Source: CAD feature listing. Evaluate the final solid. Frame: model axes, mm. A direction names the side the tool comes from. Coordinates: 2 decimals unless noted, no trailing zeros.
Item 1: Reachability of faces 1 (the flat face through (-3, -9.525, -1)), 2 (the cylindrical face through (-219.957, -9.18, 24.349)) from +Z, -Z, +X, -X, +Y, -Y: full face, straight path, thin tool, end or side. Return the list, or none.
Item 2: Line query: probe 1 along Z at (x, y) = (215, -3.75); probe 2 along X at (y, z) = (-2.75, 0) (1 decimal); probe 3 along X at (y, z) = (-4.5, 20) (3 decimals). Output: solid intervals per line, ascending.
Item 3: Pin query (flat end, axial travel): pin 1 Ø2.5 at (x, z) = (-216.5, 2.5) entering from -Y. Return the tip coordinate at first contact, or that it passes through.
```python
from build123d import *

# Parameters (mm, degrees)
RESSALTO_EXTRUS_O1_DEPTH        = 9.525
ESBO_O5_R                       = 2.78
CORTE_EXTRUS_O2_DEPTH           = 10
ESBO_O8_R                       = 2.75
CORTE_EXTRUS_O4_DEPTH           = 10
ESBO_O9_R                       = 5
CORTE_EXTRUS_O5_DEPTH           = 0.7
ESBO_O10_R                      = 5
CORTE_EXTRUS_O6_DEPTH           = 2.5
CORTE_EXTRUS_O6_DRAFT           = -45
CORTE_EXTRUS_O6_PROFILE_2_DEPTH = 2.5
CORTE_EXTRUS_O6_PROFILE_2_DRAFT = -45
CORTE_EXTRUS_O6_PROFILE_3_DEPTH = 2.5
CORTE_EXTRUS_O6_PROFILE_3_DRAFT = -45
CORTE_EXTRUS_O6_PROFILE_4_DEPTH = 2.5
CORTE_EXTRUS_O6_PROFILE_4_DRAFT = -45
CORTE_EXTRUS_O6_PROFILE_5_DEPTH = 2.5
CORTE_EXTRUS_O6_PROFILE_5_DRAFT = -45
CORTE_EXTRUS_O6_PROFILE_6_DEPTH = 2.5
CORTE_EXTRUS_O6_PROFILE_6_DRAFT = -45
ESBO_O11_R                      = 2.5
CORTE_EXTRUS_O7_DEPTH           = 10


with BuildPart() as part:
    # Esboço3 → Ressalto-extrusão1 (new body)
    with BuildSketch(Plane(origin=(0, 0, 0), x_dir=(1, 0, 0), z_dir=(0, 1, 0))):
        Polygon((-183.495, 37.21932618), (-246.505, 50), (-246.505, -50), (-183.495, -50), align=None)
        Polygon((-183.495, 50), (-183.495, 37.21932618), (183.495, -37.21932618), (183.495, 50), align=None)
        Polygon((183.495, -37.21932618), (-183.495, 37.21932618), (-183.495, -50), (183.495, -50), align=None)
        Polygon((246.505, -50), (183.495, -37.21932618), (183.495, -50), align=None)
        Polygon((183.495, 50), (183.495, -37.21932618), (246.505, -50), (246.505, 50), align=None)
        Polygon((-183.495, 50), (-246.505, 50), (-183.495, 37.21932618), align=None)
    extrude(amount=-RESSALTO_EXTRUS_O1_DEPTH)

    # Esboço5 → Corte-extrusão2 (cut)
    with BuildSketch(Plane(origin=(0, 0, 0), x_dir=(1, 0, 0), z_dir=(0, 1, 0))):
        with Locations(Location((0, -45.235, 0), (0, 0, 270))):
            Circle(ESBO_O5_R)
        with Locations(Location((-20, -45.235, 0), (0, 0, 270))):
            Circle(ESBO_O5_R)
        with Locations(Location((20, -45.235, 0), (0, 0, 270))):
            Circle(ESBO_O5_R)
        with Locations(Location((-20, 45.235, 0), (0, 0, 270))):
            Circle(ESBO_O5_R)
        with Locations(Location((20, 45.235, 0), (0, 0, 270))):
            Circle(ESBO_O5_R)
        with Locations(Location((0, 45.235, 0), (0, 0, 270))):
            Circle(ESBO_O5_R)
    extrude(amount=-CORTE_EXTRUS_O2_DEPTH, mode=Mode.SUBTRACT)

    # Esboço8 → Corte-extrusão4 (cut)
    with BuildSketch(Plane.XZ.offset(9.525)):
        with Locations(Location((-188.84, 19.950903247, 0), (0, 0, 270))):
            Circle(ESBO_O8_R)
        with Locations(Location((-188.84, -19.95, 0), (0, 0, 270))):
            Circle(ESBO_O8_R)
        with Locations(Location((-241.16, 19.950903247, 0), (0, 0, 270))):
            Circle(ESBO_O8_R)
        with Locations(Location((-241.16, -19.95, 0), (0, 0, 270))):
            Circle(ESBO_O8_R)
        with Locations(Location((241.16, -19.95, 0), (0, 0, 90))):
            Circle(ESBO_O8_R)
        with Locations(Location((241.16, 19.950903247, 0), (0, 0, 90))):
            Circle(ESBO_O8_R)
        with Locations(Location((188.84, -19.95, 0), (0, 0, 90))):
            Circle(ESBO_O8_R)
        with Locations(Location((188.84, 19.950903247, 0), (0, 0, 90))):
            Circle(ESBO_O8_R)
    extrude(amount=-CORTE_EXTRUS_O4_DEPTH, mode=Mode.SUBTRACT)

    # Esboço9 → Corte-extrusão5 (cut)
    with BuildSketch(Plane.XZ.offset(9.525)):
        with Locations(Location((215, 25, 0), (0, 0, 270))):
            Circle(ESBO_O9_R)
        with Locations(Location((215, 0, 0), (0, 0, 270))):
            Circle(ESBO_O9_R)
        with Locations(Location((215, -25, 0), (0, 0, 270))):
            Circle(ESBO_O9_R)
        with Locations(Location((-215, -25, 0), (0, 0, 90))):
            Circle(ESBO_O9_R)
        with Locations(Location((-215, 0, 0), (0, 0, 90))):
            Circle(ESBO_O9_R)
        with Locations(Location((-215, 25, 0), (0, 0, 90))):
            Circle(ESBO_O9_R)
    extrude(amount=-CORTE_EXTRUS_O5_DEPTH, mode=Mode.SUBTRACT)


with BuildPart() as corte_extrus_o6_tool:
    # Esboço10 → Corte-extrusão6 (with draft: the straight prism first)
    with BuildSketch(Plane.XZ.offset(8.825)):
        with Locations(Location((215, 25, 0), (0, 0, 270))):
            Circle(ESBO_O10_R)
    extrude(amount=-CORTE_EXTRUS_O6_DEPTH)
    # Corte-extrusão6: the draft: its side faces are tilted about the plane it starts from
    corte_extrus_o6_sides = [corte_extrus_o6_tool.faces().sort_by_distance(p)[0] for p in [
        (215, -7.575, 30),
    ]]
    draft(corte_extrus_o6_sides, Plane.XZ.offset(8.825), CORTE_EXTRUS_O6_DRAFT)


with BuildPart() as part_1:
    add(part.part)

    # Corte-extrusão6: cut by corte_extrus_o6_tool
    add(corte_extrus_o6_tool.part, mode=Mode.SUBTRACT)


with BuildPart() as corte_extrus_o6_profile_2_tool:
    # Esboço10 → Corte-extrusão6 profile 2 (with draft: the straight prism first)
    with BuildSketch(Plane.XZ.offset(8.825)):
        with Locations((214.7625, 0)):
            Circle(ESBO_O10_R)
    extrude(amount=-CORTE_EXTRUS_O6_PROFILE_2_DEPTH)
    # Corte-extrusão6 profile 2: the draft: its side faces are tilted about the plane it starts from
    corte_extrus_o6_profile_2_sides = [corte_extrus_o6_profile_2_tool.faces().sort_by_distance(p)[0] for p in [
        (209.7625, -7.575, 0),
    ]]
    draft(corte_extrus_o6_profile_2_sides, Plane.XZ.offset(8.825), CORTE_EXTRUS_O6_PROFILE_2_DRAFT)


with BuildPart() as part_2:
    add(part_1.part)

    # Corte-extrusão6 profile 2: cut by corte_extrus_o6_profile_2_tool
    add(corte_extrus_o6_profile_2_tool.part, mode=Mode.SUBTRACT)


with BuildPart() as corte_extrus_o6_profile_3_tool:
    # Esboço10 → Corte-extrusão6 profile 3 (with draft: the straight prism first)
    with BuildSketch(Plane.XZ.offset(8.825)):
        with Locations(Location((215, -25, 0), (0, 0, 270))):
            Circle(ESBO_O10_R)
    extrude(amount=-CORTE_EXTRUS_O6_PROFILE_3_DEPTH)
    # Corte-extrusão6 profile 3: the draft: its side faces are tilted about the plane it starts from
    corte_extrus_o6_profile_3_sides = [corte_extrus_o6_profile_3_tool.faces().sort_by_distance(p)[0] for p in [
        (215, -7.575, -20),
    ]]
    draft(corte_extrus_o6_profile_3_sides, Plane.XZ.offset(8.825), CORTE_EXTRUS_O6_PROFILE_3_DRAFT)


with BuildPart() as part_3:
    add(part_2.part)

    # Corte-extrusão6 profile 3: cut by corte_extrus_o6_profile_3_tool
    add(corte_extrus_o6_profile_3_tool.part, mode=Mode.SUBTRACT)


with BuildPart() as corte_extrus_o6_profile_4_tool:
    # Esboço10 → Corte-extrusão6 profile 4 (with draft: the straight prism first)
    with BuildSketch(Plane.XZ.offset(8.825)):
        with Locations(Location((-215, -25, 0), (0, 0, 90))):
            Circle(ESBO_O10_R)
    extrude(amount=-CORTE_EXTRUS_O6_PROFILE_4_DEPTH)
    # Corte-extrusão6 profile 4: the draft: its side faces are tilted about the plane it starts from
    corte_extrus_o6_profile_4_sides = [corte_extrus_o6_profile_4_tool.faces().sort_by_distance(p)[0] for p in [
        (-215, -7.575, -30),
    ]]
    draft(corte_extrus_o6_profile_4_sides, Plane.XZ.offset(8.825), CORTE_EXTRUS_O6_PROFILE_4_DRAFT)


with BuildPart() as part_4:
    add(part_3.part)

    # Corte-extrusão6 profile 4: cut by corte_extrus_o6_profile_4_tool
    add(corte_extrus_o6_profile_4_tool.part, mode=Mode.SUBTRACT)


with BuildPart() as corte_extrus_o6_profile_5_tool:
    # Esboço10 → Corte-extrusão6 profile 5 (with draft: the straight prism first)
    with BuildSketch(Plane.XZ.offset(8.825)):
        with Locations((-214.7625, 0)):
            Circle(ESBO_O10_R)
    extrude(amount=-CORTE_EXTRUS_O6_PROFILE_5_DEPTH)
    # Corte-extrusão6 profile 5: the draft: its side faces are tilted about the plane it starts from
    corte_extrus_o6_profile_5_sides = [corte_extrus_o6_profile_5_tool.faces().sort_by_distance(p)[0] for p in [
        (-219.7625, -7.575, 0),
    ]]
    draft(corte_extrus_o6_profile_5_sides, Plane.XZ.offset(8.825), CORTE_EXTRUS_O6_PROFILE_5_DRAFT)


with BuildPart() as part_5:
    add(part_4.part)

    # Corte-extrusão6 profile 5: cut by corte_extrus_o6_profile_5_tool
    add(corte_extrus_o6_profile_5_tool.part, mode=Mode.SUBTRACT)


with BuildPart() as corte_extrus_o6_profile_6_tool:
    # Esboço10 → Corte-extrusão6 profile 6 (with draft: the straight prism first)
    with BuildSketch(Plane.XZ.offset(8.825)):
        with Locations(Location((-215, 25, 0), (0, 0, 90))):
            Circle(ESBO_O10_R)
    extrude(amount=-CORTE_EXTRUS_O6_PROFILE_6_DEPTH)
    # Corte-extrusão6 profile 6: the draft: its side faces are tilted about the plane it starts from
    corte_extrus_o6_profile_6_sides = [corte_extrus_o6_profile_6_tool.faces().sort_by_distance(p)[0] for p in [
        (-215, -7.575, 20),
    ]]
    draft(corte_extrus_o6_profile_6_sides, Plane.XZ.offset(8.825), CORTE_EXTRUS_O6_PROFILE_6_DRAFT)


with BuildPart() as part_6:
    add(part_5.part)

    # Corte-extrusão6 profile 6: cut by corte_extrus_o6_profile_6_tool
    add(corte_extrus_o6_profile_6_tool.part, mode=Mode.SUBTRACT)

    # Esboço11 → Corte-extrusão7 (cut)
    with BuildSketch(Plane.XZ.offset(9.525)):
        with Locations(Location((215, 25, 0), (0, 0, 270))):
            Circle(ESBO_O11_R)
        with Locations(Location((214.7625, 0, 0), (0, 0, 270))):
            Circle(ESBO_O11_R)
        with Locations(Location((215, -25, 0), (0, 0, 270))):
            Circle(ESBO_O11_R)
        with Locations(Location((-215, -25, 0), (0, 0, 90))):
            Circle(ESBO_O11_R)
        with Locations(Location((-214.7625, 0, 0), (0, 0, 90))):
            Circle(ESBO_O11_R)
        with Locations(Location((-215, 25, 0), (0, 0, 90))):
            Circle(ESBO_O11_R)
    extrude(amount=-CORTE_EXTRUS_O7_DEPTH, mode=Mode.SUBTRACT)


solid = part_6.part
```
Verdict:
1. face 1: +Z, -Z, +X, -X, -Y
1. face 2: -Y
2. probe 1: z = -50 to -27.5, -22.5 to -2.49, 2.49 to 22.5, 27.5 to 50
2. probe 2: x = -246.5 to -217.3, -212.3 to 212.3, 217.3 to 246.5
2. probe 3: x = -246.505 to -243.91, -238.41 to -191.59, -186.09 to 186.09, 191.59 to 238.41, 243.91 to 246.505
3. pin 1: stops at y = -8.12
